Can you work these out from the model? Positions are in its coordinate system, mm. Face numbers are marked on the shaded views. A direction names the side the tool comes from. Round coordinates to 2 decimals unless told otherwise and drop trailing zeros. Loops run counter-clockwise (first coordinate to the right, second up) from the corner with the lowest first, then second, coordinate; pieces in that order, holes last. Notation, with made-up numbers: (-13.75, -39.75) -> (-3.75, -39.75) arc R24 ccw to (-3.75, -29.75) -> close; hole circle Ø7 at (84, 26). An arc over 180 degrees is marked (long way). Write each question's results on one line, items separated by ' | '.
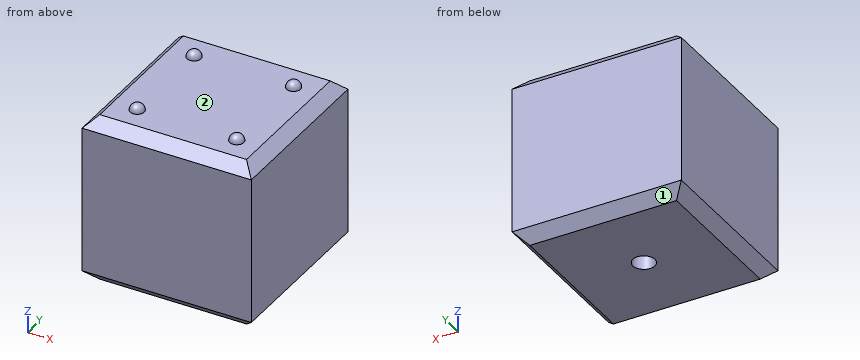
from build123d import *

# Parameters (mm, degrees)
F0_W     = 76.2
F0_H     = 76.2
F1_DEPTH = 76.2
F2_SIZE  = 5.08
F3_R     = 4.953
F4_DEPTH = 25.4
F5_R     = 3.175
F6_DEPTH = 3.175
F7_R     = 3.17499


# Not quite as in the source:
# - a fillet or chamfer is up to 0.001 mm smaller than in the source, because OpenCascade refuses the exact size


with BuildPart() as f1:
    # F0 (on Top) → F1 (new body)
    with BuildSketch(Plane.XY):
        with Locations((-0.4966171047, -21.9681663439)):
            Rectangle(F0_W, F0_H)
    extrude(amount=F1_DEPTH)

    # F2
    f2_edges = [f1.edges().sort_by_distance(p)[0] for p in [
        (-0.496617, -60.068166, 76.2),
        (37.603383, -21.968166, 76.2),
        (-0.496617, 16.131834, 76.2),
        (-38.596617, -21.968166, 76.2),
        (37.603383, -21.968166, 0),
        (-0.496617, -60.068166, 0),
        (-38.596617, -21.968166, 0),
        (-0.496617, 16.131834, 0),
    ]]
    chamfer(f2_edges, length=F2_SIZE)

    # F3 (on face) → F4 (cut)
    with BuildSketch(Plane(origin=(0, 0, 0), x_dir=(1, 0, 0), z_dir=(0, 0, -1))):
        with Locations((0, 21.9681663439)):
            Circle(F3_R)
    extrude(amount=-F4_DEPTH, mode=Mode.SUBTRACT)

    # F5 (on face) → F6 (join)
    with BuildSketch(Plane.XY.offset(76.2)):
        with Locations((-22.4647834486, 0)):
            Circle(F5_R)
        with Locations((22.3648820278, 0)):
            Circle(F5_R)
        with Locations((-22.4647834486, -44.8296654764)):
            Circle(F5_R)
        with Locations((22.3648820278, -44.8296654764)):
            Circle(F5_R)
    extrude(amount=F6_DEPTH)

    # F7 (radius 3.175 in the source; OpenCascade refuses exactly that, so slightly less here)
    f7_edges = [f1.edges().sort_by_distance(p)[0] for p in [
        (-25.639783, -44.829665, 79.375),
        (-25.639783, 0, 79.375),
        (19.189882, 0, 79.375),
        (19.189882, -44.829665, 79.375),
    ]]
    fillet(f7_edges, radius=F7_R)


solid = f1.part
1. If we section it at B-B (y = -7): List the corners of the cut face in (x, z) for me.
Final values:
outline: (-38.6, 5.08) -> (-33.52, 0) -> (32.52, 0) -> (37.6, 5.08) -> (37.6, 71.12) -> (32.52, 76.2) -> (-33.52, 76.2) -> (-38.6, 71.12) -> close
2. Please list where these lines run through material, in increasing order: line 1 (Y direction, x = 0, z = 6.75); line 2 (Z direction, x = -13, y = -3); line 3 (X direction, y = -25, z = 13). Write a range as from..to.
Final values:
line 1: -60.07..-26.92, -17.02..16.13 | line 2: 0..76.2 | line 3: -38.6..-3.92, 3.92..37.6
3. If we section it at C-C (x = 0): List the corners of the cut face in (y, z) for me.
Final values:
outline: (-60.07, 5.08) -> (-54.99, 0) -> (-26.92, 0) -> (-26.92, 25.4) -> (-17.02, 25.4) -> (-17.02, 0) -> (11.05, 0) -> (16.13, 5.08) -> (16.13, 71.12) -> (11.05, 76.2) -> (-54.99, 76.2) -> (-60.07, 71.12) -> close
4. Will this pin go through, and if not, where does the flat tip stop? pin 1 (2 mm diameter, centred on x = 5, y = -46.5, fed in from +Z).
Final values:
pin 1: z = 76.2
5. On a 3-axis mill with a long thin cutter (end or side, diameter ignored), from which of +Z, -Z, +X, -X, +Y, -Y can I reach the whole of each face in a straight line? I mean the marked faces 1 and 2. Say none if no direction works.
Final values:
face 1: -Z, +X, -X, +Y | face 2: +Z
6. If we section it at A-A (x = 30): List the corners of the cut face in (y, z) for me.
Final values:
outline: (-60.07, 5.08) -> (-54.99, 0) -> (11.05, 0) -> (16.13, 5.08) -> (16.13, 71.12) -> (11.05, 76.2) -> (-54.99, 76.2) -> (-60.07, 71.12) -> close
